Verification items for the finished model (mm, model axes). Give positions to 0.01 mm unless a question says otherwise; leave off trailing zeros. Order: outer loops, then holes, each group sorted by start corner. A loop starts at its lowest first (then second) coordinate and runs counter-clockwise, first axis right, second up. Notation, with made-up numbers: (-31.75, 8.25) -> (-9.75, 8.25) arc R20 cw to (-9.75, 35.25) -> close; hole circle Ø3 at (-24.5, -33). An arc over 180 degrees is marked (long way). One line per question, with ' | ' between items. Start each with the question number.
Q1. Section check A-A on z = 0.7. Give the number of separate pieces and of enclosed holes in the cut face, plus the area to 3 significant figures.
Q2. Section check B-B on x = -30.5. Record the cut outline in (y, z).
Q3. Material ranges on probe 1 along Y at (x, z) = (-15.5, 1.1); probe 2 along Y at (x, z) = (-36, 0.95); probe 3 along Y at (x, z) = (-17.5, 1.3), recorded low to high. Write a range as [from, to].
Q4. Go/stop test with a flat-tipped pin: pin 1 (0.8 mm diameter, centred on x = 47, z = 0.5, fed in from +Y). Record where the tip stops, or that it passes through.
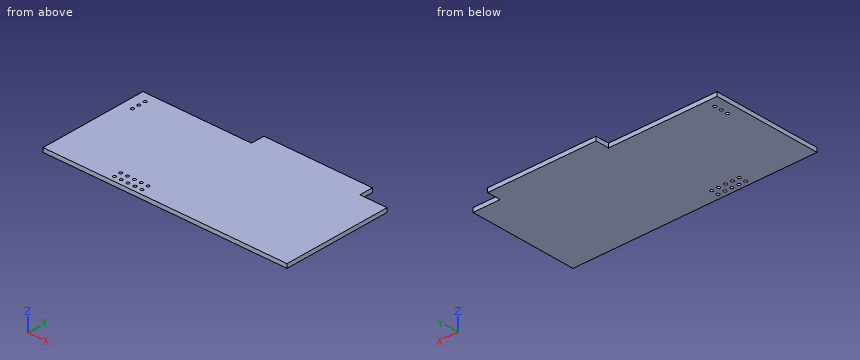
from build123d import *

# Parameters (mm, degrees)
EXTRUDE_1_DEPTH     = 1.5
SKETCH_2_R          = 0.55
CUT_EXTRUDE_1_DEPTH = 1.5


with BuildPart() as part:
    # Эскиз1 → Вытянуть1 (new body)
    with BuildSketch(Plane.XY):
        Polygon((0, 20), (0, 25), (40, 25), (40, 20), (50, 20), (50, -20), (-40, -20), (-40, 20), align=None)
    extrude(amount=EXTRUDE_1_DEPTH)

    # Эскиз2 → Вырез-Вытянуть1 (cut)
    with BuildSketch(Plane.XY.offset(1.5)):
        with Locations((-36, 16.54)):
            Circle(SKETCH_2_R)
        with Locations((-36, 11.46)):
            Circle(SKETCH_2_R)
        with Locations((-36, 14)):
            Circle(SKETCH_2_R)
        with Locations((-15.5, -15.5)):
            Circle(SKETCH_2_R)
        with Locations((-15.5, -18.04)):
            Circle(SKETCH_2_R)
        with Locations((-12.96, -15.5)):
            Circle(SKETCH_2_R)
        with Locations((-12.96, -18.04)):
            Circle(SKETCH_2_R)
        with Locations((-10.42, -15.5)):
            Circle(SKETCH_2_R)
        with Locations((-10.42, -18.04)):
            Circle(SKETCH_2_R)
        with Locations((-7.88, -15.5)):
            Circle(SKETCH_2_R)
        with Locations((-7.88, -18.04)):
            Circle(SKETCH_2_R)
        with Locations((-5.34, -15.5)):
            Circle(SKETCH_2_R)
        with Locations((-5.34, -18.04)):
            Circle(SKETCH_2_R)
    extrude(amount=-CUT_EXTRUDE_1_DEPTH, mode=Mode.SUBTRACT)


solid = part.part
Filled in:
1) separate pieces: 1 | enclosed holes: 13 | area: 3,790 mm²
2) outline: (-20, 0) -> (20, 0) -> (20, 1.5) -> (-20, 1.5) -> close
3) probe 1: [-20, -18.59], [-17.49, -16.05], [-14.95, 20] | probe 2: [-20, 10.91], [12.01, 13.45], [14.55, 15.99], [17.09, 20] | probe 3: [-20, 20]
4) pin 1: y = 20
